For this review, take the finished solid that the model builds, in its own axes (mm). A direction names the side the tool comes from. Coordinates: 2 decimals unless noted, no trailing zeros. Loops run counter-clockwise (first coordinate to the right, second up) from the corner with the lowest first, then second, coordinate; pieces in that order, holes last. Notation, with made-up numbers: (-6, -12.5) -> (7, -12.5) arc R24 cw to (7, -0.5) -> close; hole circle Ø6 at (72.25, 27.25). An arc over 180 degrees is marked (long way). Answer in a Markdown table with one row per item.
Autodesk Inventor part; units mm, degrees
ref_plane "YZ Plane" through (0, 0, 0) normal (1, 0, 0) x (0, 1, 0)
ref_plane "XZ Plane" through (0, 0, 0) normal (0, 1, 0) x (-1, 0, 0)
ref_plane "XY Plane" through (0, 0, 0) normal (0, 0, 1) x (1, 0, 0)
sketch "Esquisse1" plane through (0, 0, 0) normal (1, 0, 0) x (0, 1, 0)
  line L0 (21, 21) -> (-21, 21)
  line L1 (-21, 21) -> (-21, -21)
  line L2 (-21, -21) -> (21, -21)
  line L3 (21, -21) -> (21, 21)
  line L4 (21, 21) -> (-21, -21)
  line L5 (-21, 21) -> (21, -21)
  circle A0 centre (0, 0) radius 11
  line L6 (15.5, 15.5) -> (-15.5, 15.5)
  line L7 (-15.5, 15.5) -> (-15.5, -15.5)
  line L8 (-15.5, -15.5) -> (15.5, -15.5)
  line L9 (15.5, -15.5) -> (15.5, 15.5)
  line L10 (15.5, 15.5) -> (-15.5, -15.5)
  line L11 (-15.5, 15.5) -> (15.5, -15.5)
  circle A1 centre (15.5, 15.5) radius 1.75
  circle A2 centre (-15.5, 15.5) radius 1.75
  line L12 (21, 0) -> (-21, 0)
  circle A3 centre (15.5, -15.5) radius 1.75
  circle A4 centre (-15.5, -15.5) radius 1.75
  point P0 (0, 0)
  point P1 (0, 0)
  dimension "d0" = 42
  dimension "d1" = 22
  dimension "d2" = 31
  dimension "d3" = 3.5
  dimension "d4" = 3.5
extrude "Extrusion1" add sketch "Esquisse1" along normal blind 10 contours L4 A1 L6 A2 L5 L0 | L3 L12 L9 A1 L4 | L5 A2 L7 L12 L1 | L3 L5 A3 L9 L12 | L12 L7 A4 L4 L1 | L2 L4 A4 L8 A3 L5 | L12 A0 L4 A1 L9 | L9 A3 L5 A0 L12 | A1 L4 A0 L5 A2 L6 | L12 A0 L4 A4 L7 | L7 A2 L5 A0 L12 | L8 A4 L4 A0 L5 A3
sketch "Esquisse2" plane through (0, -21, -21) normal (0, -1, 0) x (1, 0, 0)
  point P0 (0, 21)
sketch "Esquisse3" plane through (0, -21, -21) normal (0, -1, 0) x (1, 0, 0)
  line L0 (0, 42) -> (0, 0)
  line L1 (0, 42) -> (12, 42)
  line L2 (12, 42) -> (12, 0)
  line L3 (12, 0) -> (0, 0)
  line L4 (0, 0) -> (0, 42)
  point P0 (0, 21)
  dimension "d19" = 12
extrude "Extrusion2" add sketch "Esquisse3" along normal blind 10
sketch "Esquisse4" plane through (10, 0, 0) normal (1, 0, 0) x (0, 0, -1)
  line L0 (21, -31) -> (-21, -31)
  line L1 (21, 21) -> (21, -31)
  line L2 (-21, -31) -> (21, -31)
  line L3 (21, -31) -> (21, -21)
  line L4 (21, -21) -> (-21, -21)
  line L5 (-21, -21) -> (-21, -31)
  point P0 (0, 0)
extrude "Extrusion3" add sketch "Esquisse4" along normal blind 8
sketch "Esquisse5" plane through (18, 0, 0) normal (1, 0, 0) x (0, 0, -1)
  line L0 (-21, -21) -> (-21, -31)
  line L1 (-21, -31) -> (21, -31)
  line L2 (-21, -21) -> (21, -21)
  line L3 (21, -21) -> (21, -31)
  line L4 (21, -31) -> (-21, -31)
  line L5 (-21, -31) -> (-21, -21)
  point P0 (0, 0)
extrude "Extrusion4" add sketch "Esquisse5" along normal blind 40
sketch "Esquisse9" plane through (10, -21, 21) normal (0, 1, 0) x (1, 0, 0)
  line L0 (0, 0) -> (0, 42)
  line L1 (0, 0) -> (48, 0)
  line L2 (0, 42) -> (8, 42)
  line L3 (8, 42) -> (8, 0)
  line L4 (8, 0) -> (0, 0)
  line L5 (0, 0) -> (0, 42)
  line L6 (0, 21) -> (8, 21)
  line L7 (0, 29) -> (8, 29)
  line L8 (8, 29) -> (8, 13)
  line L9 (8, 13) -> (0, 13)
  line L10 (0, 13) -> (0, 29)
  point P0 (-10, 21)
  point P1 (0, 13)
  point P2 (8, 29)
  dimension "d24" = 16
extrude "Extrusion7" cut sketch "Esquisse9" against normal blind 10 contours L0 L9 L3 L1 | L0 L2 L3 L7
sketch "Esquisse10" plane through (0, 0, 0) normal (-1, 0, 0) x (0, 0, 1)
  line L0 (21, 21) -> (21, -31)
  line L1 (-21, -31) -> (21, -31)
  line L2 (21, -31) -> (21, -21)
  line L3 (21, -21) -> (-21, -21)
  line L4 (-21, -21) -> (-21, -31)
  point P0 (0, 0)
  point P1 (21, -31)
extrude "Extrusion8" add sketch "Esquisse10" along normal blind 30
sketch "Esquisse11" plane through (0, -31, -21) normal (0, -1, 0) x (1, 0, 0)
  line L0 (18, 42) -> (58, 42)
  line L1 (18, 0) -> (58, 0)
  line L2 (0, 42) -> (-30, 42)
  line L3 (10, 29) -> (18, 29)
  line L4 (14, 29) -> (14, 13)
  line L5 (18, 13) -> (10, 13)
  circle A0 centre (-11, 21) radius 4.05
  circle A1 centre (39, 21) radius 4.05
  point P0 (0, 21)
  point P1 (0, 0)
  point P2 (33, 21)
  point P3 (0, 21)
  point P4 (14, 21)
  dimension "d32" = 8.1
  dimension "d33" = 25
extrude "Extrusion9" cut sketch "Esquisse11" against normal blind 8
sketch "Esquisse12" plane through (0, -31, -21) normal (0, -1, 0) x (1, 0, 0)
  line L0 (0, 42) -> (-30, 42)
  line L1 (-30, 42) -> (10, 42)
  line L2 (10, 42) -> (10, 29)
  line L3 (18, 29) -> (10, 29)
  line L4 (18, 42) -> (18, 29)
  line L5 (18, 29) -> (18, 42)
  line L6 (18, 42) -> (48, 42)
  line L7 (48, 0) -> (18, 0)
  line L8 (18, 0) -> (18, 13)
  line L9 (18, 13) -> (10, 13)
  line L10 (10, 13) -> (10, 0)
  line L11 (-30, 0) -> (-30, 42)
  line L12 (10, 29) -> (18, 29)
  line L13 (10, 13) -> (18, 13)
  line L14 (0, 0) -> (10, 0)
  line L15 (0, 0) -> (10.2767, 0)
  line L16 (0, 0) -> (10, 0)
  line L17 (0, 0) -> (-30, 0)
  line L18 (-30, 0) -> (0, 0)
  circle A0 centre (-11, 21) radius 4.05
  circle A1 centre (39, 21) radius 4.05
  line L19 (18, 42) -> (58, 42)
  line L20 (48, 42) -> (58, 42)
  line L21 (58, 42) -> (58, 0)
  line L22 (18, 0) -> (58, 0)
  line L23 (48, 0) -> (58, 0)
  point P0 (0, 21)
extrude "Extrusion10" add sketch "Esquisse12" along normal blind 5
sketch "Esquisse13" plane through (0, 0, 0) normal (-1, 0, 0) x (0, 0, 1)
  circle A0 centre (-15.5, 15.5) radius 1.75
  circle A1 centre (-15.5, 15.5) radius 1.75
  circle A2 centre (15.5, 15.5) radius 1.75
  circle A3 centre (15.5, 15.5) radius 1.75
  circle A4 centre (15.5, -15.5) radius 1.75
  circle A5 centre (15.5, -15.5) radius 1.75
  circle A6 centre (-15.5, -15.5) radius 1.75
  circle A7 centre (-15.5, -15.5) radius 1.75
  line L0 (-21, -21) -> (21, -21)
  line L1 (-21, 21) -> (21, 21)
  line L2 (21, 21) -> (21, -21)
  line L3 (21, -21) -> (-21, -21)
  line L4 (-21, -21) -> (-21, 21)
  circle A8 centre (0, 0) radius 11
extrude "Extrusion11" cut sketch "Esquisse13" against normal blind 0.5
fillet "Congé5" radius 21 4 edges at (-30, -28.5, 21) (-30, -28.5, -21) (58, -28.5, -21) (58, -28.5, 21)
fillet "Congé6" radius 5 2 edges at (5.25, 21, -21) (5.25, 21, 21)
fillet "Congé7" radius 5 4 edges at (14, -21, -8) (14, -21, 8) (14, -36, 8) (14, -36, -8)
fillet "Congé8" radius 1 2 edges at (34.95, -36, 0) (-15.05, -36, 0)
properties part number "tete_Impression 3D"
Item 1: Take a section at C-C, the plane y = 8. State the section outline as (x, z) points.
Worked answers:
| item | result |
|---|---|
| outline | (0.5, -21) -> (10, -21) -> (10, -7.55) -> (0.5, -7.55) -> close; (0.5, 7.55) -> (10, 7.55) -> (10, 21) -> (0.5, 21) -> close |
Item 2: For L1, parallel to Z at x = 6, y = -15.5; L2, parallel to Z at x = 4.75, y = 0; L3, parallel to X at y = -26.5, z = 3, list the stretches that pass through material, from the lowest coordinate up.
Worked answers:
| item | result |
|---|---|
| L1 | -21 to -17.25, -13.75 to 13.75, 17.25 to 21 |
| L2 | -21 to -11, 11 to 21 |
| L3 | -29.78 to -13.72, -8.28 to 36.28, 41.72 to 57.78 |
Item 3: For faces 4 (the flat face through (14, -28, -8)), 5 (the flat face through (0.5, -9, 9)), 6 (the cylindrical face through (14, -23, 7)), list the 3-axis set-ups (+Z, -Z, +X, -X, +Y, -Y) from which the entire face can be reached by the end or side of a thin tool; tool diameter is ignored.
Worked answers:
| item | result |
|---|---|
| face 4 | -Z, +Y, -Y |
| face 5 | +Z, -Z, -X, +Y |
| face 6 | +Z, +Y |
Item 4: Insertion check: pin 1 (4 mm diameter, centred on y = 15.5, z = -15.5, fed in from +X); pin 2 (16.5 mm diameter, centred on y = -30, z = 11.5, fed in from -X); pin 3 (5 mm diameter, centred on x = -11, z = 0, fed in from +Y). Each pin has a flat end and moves straight along its axis. Give the tip position at first contact, or say it passes through.
Worked answers:
| item | result |
|---|---|
| pin 1 | x = 10 |
| pin 2 | x = -29.75 |
| pin 3 | y = -21 |
Item 5: Take a section at D-D, the plane x = 39. State the section outline as (y, z) points, and give its area (3 significant figures).
Worked answers:
| item | result |
|---|---|
| outline | (-36, -20.9) -> (-21, -20.9) -> (-21, 20.9) -> (-36, 20.9) -> (-36, 5.05) arc R1 ccw to (-35, 4.05) -> (-23, 4.05) -> (-23, -4.05) -> (-35, -4.05) arc R1 ccw to (-36, -5.05) -> close |
| area | 521 mm² |
Item 6: Take a section at A-A, the plane x = 14. State the section outline as (y, z) points.
Worked answers:
| item | result |
|---|---|
| outline | (-36, -3) arc R5 ccw to (-31, -8) -> (-26, -8) arc R5 ccw to (-21, -3) -> (-21, 3) arc R5 ccw to (-26, 8) -> (-31, 8) arc R5 ccw to (-36, 3) -> close |
Item 7: Take a section at B-B, the plane x = 2. State the section outline as (y, z) points.
Worked answers:
| item | result |
|---|---|
| outline | (-36, -21) -> (16, -21) arc R5 ccw to (21, -16) -> (21, 16) arc R5 ccw to (16, 21) -> (-36, 21) -> close; hole circle Ø3.5 at (-15.5, -15.5); hole circle Ø3.5 at (-15.5, 15.5); hole circle Ø22 at (0, 0); hole circle Ø3.5 at (15.5, -15.5); hole circle Ø3.5 at (15.5, 15.5) |
Item 8: The part is to be moulded in two halves that separate along Y. For faces 1 (the flat face through (-11, -23, 0)), 2 (the cylindrical face through (5.184, 15.272, -17.235)), 3 (the cylindrical face through (14, -23, -7)), say which applies: +Y half, -Y half, draft (parallel to the pull), parting line (faces both ways), or undercut.
Worked answers:
| item | result |
|---|---|
| face 1 | -Y half |
| face 2 | undercut |
| face 3 | +Y half |
